```python
from build123d import *

# Parameters (mm, degrees)
SKETCH_W     = 12
SKETCH_H     = 12
SKETCH_R     = 4
PAD_DEPTH    = 12
SKETCH001_R  = 4
POCKET_DEPTH = 12.001


with BuildPart() as part:
    # Sketch → Pad (new body)
    with BuildSketch(Plane.XY):
        with Locations((6, 6)):
            Rectangle(SKETCH_W, SKETCH_H)
        with Locations((6, 6)):
            Circle(SKETCH_R, mode=Mode.SUBTRACT)
    extrude(amount=PAD_DEPTH)

    # Sketch001 (on Face1 of Pad) → Pocket (cut, through all)
    with BuildSketch(Plane.XZ):
        with Locations((6, 6)):
            Circle(SKETCH001_R)
    extrude(amount=-POCKET_DEPTH, mode=Mode.SUBTRACT)


solid = part.part
```
CAD build for the part. Positions are in the model's coordinates, mm. Coordinates: 2 decimals unless noted, no trailing zeros. Order: outer loops, then holes, each group sorted by start corner. A loop starts at its lowest first (then second) coordinate and runs counter-clockwise, first axis right, second up. Notation, with made-up numbers: (6.25, -18.5) - (56.25, -18.5) arc R4 cw to (56.25, -13.5) - close; hole circle Ø2 at (0.5, 37). An arc over 180 degrees is marked (long way). Answer in a Markdown table with one row per item.
1. Flat gauge pin, fed straight in: P1, Ø6.5, axis at x = 6, z = 6, coming from the +Y side. Where does the tip first touch, or does it go through?
Answer:
| item | result |
|---|---|
| P1 | through |
2. Pull direction X, two halves, no side cores. Call faces 1 (the face through (1.9, 0, 4.6)), 2 (the face through (2, 6, 10)), 3 (the face through (0, 6, 6)), 4 (the face through (2, 10, 6)): +X half, -X half, draft (parallel to the pull), parting line (faces both ways), or undercut.
Answer:
| item | result |
|---|---|
| face 1 | draft |
| face 2 | undercut |
| face 3 | -X half |
| face 4 | undercut |
3. Slice it at A-A, the plane x = 6. List the corners of the cut face in (y, z), then the cut area to 3 significant figures.
Answer:
| item | result |
|---|---|
| outline | (0, 0) - (2, 0) - (2, 2) - (0, 2) - close; (0, 10) - (2, 10) - (2, 12) - (0, 12) - close; (10, 0) - (12, 0) - (12, 2) - (10, 2) - close; (10, 10) - (12, 10) - (12, 12) - (10, 12) - close |
| area | 16.0 mm² |
4. Slice it at C-C, the plane z = 9.5. List the corners of the cut face in (x, y), then the cut area to 3 significant figures.
Answer:
| item | result |
|---|---|
| outline | (0, 0) - (4.06, 0) - (4.06, 2.5) arc R4 cw to (4.06, 9.5) - (4.06, 12) - (0, 12) - close; (7.94, 0) - (12, 0) - (12, 12) - (7.94, 12) - (7.94, 9.5) arc R4 cw to (7.94, 2.5) - close |
| area | 77.0 mm² |
5. Slice it at D-D, the plane y = 4. List the corners of the cut face in (x, z).
Answer:
| item | result |
|---|---|
| outline | (0, 0) - (2.54, 0) - (2.54, 4) arc R4 cw to (2.54, 8) - (2.54, 12) - (0, 12) - close; (9.46, 0) - (12, 0) - (12, 12) - (9.46, 12) - (9.46, 8) arc R4 cw to (9.46, 4) - close |
6. Drill centre lines: L1, parallel to X at y = 7.5, z = 6; L2, parallel to Y at x = 3.5, z = 1.5. Where is each one in solid material? Low to high. Write a range as from..to.
Answer:
| item | result |
|---|---|
| L1 | 0..2, 10..12 |
| L2 | 0..2.88, 9.12..12 |
7. Slice it at B-B, the plane y = 1. List the corners of the cut face in (x, z), then the cut area to 3 significant figures.
Answer:
| item | result |
|---|---|
| outline | (0, 0) - (12, 0) - (12, 12) - (0, 12) - close; hole circle Ø8 at (6, 6) |
| area | 93.7 mm² |
